Check sheet for the modelled part. Datum: model origin and axes. Units: mm. A direction names the side the tool comes from. Round coordinates to 2 decimals unless told otherwise and drop trailing zeros. Write each loop counter-clockwise with the first axis right and the second up, starting at its lowest first coordinate (ties: lowest second). Pieces come first, ordered by that corner, then holes. Notation, with made-up numbers: (-4, 33.25) - (42, 33.25) arc R21 ccw to (42, 67.25) - close; hole circle Ø11 at (85, 65.5). An arc over 180 degrees is marked (long way). Answer as a JSON object with one key per item and string values. Group by question number.
Item 1: Set-up check for faces 1 (the flat face through (-1.22, 0.49, -0.87)), 2 (the flat face through (0, 2, 0)), 3 (the cylindrical face through (-0.862, -0.596, 2.685)): record each of +Z, -Z, +X, -X, +Y, -Y from which the full face is reachable in a straight line by a thin tool's end or side.
Item 2: Sectioned sample at A-A on x = 5.75. Record the boundary of the cut face in (y, z), plus the area to 3 significant figures.
Item 3: Thickness scan on line 1 (X direction, y = 1.8, z = -0.9); line 2 (Z direction, x = -0.75, y = -0.5); line 3 (Y direction, x = 7.75, z = -1.15). Record the ranges inside material, lowest first.
Item 4: Release check for a two-part mould opening along Y. For faces 4 (the flat face through (10, 0, 0)), 5 (the flat face through (-1, -1, 0)), 6 (the cylindrical face through (4.83, -1.5, -0.07)) record: pulls with the +Y half, pulls with the -Y half, needs draft (parallel to the pull), parting line crosses it, or undercut.
Item 5: Gauge pin test, flat end, axial feed: P1, Ø3, axis at x = 3, z = -1, coming from the -Y side. Record the tip position at first contact, or that the pin passes through.
Autodesk Inventor part; units mm, degrees
ref_plane "Work Plane1" through (29, 0, 0) normal (0, -1, 0) x (1, 0, 0)
ref_plane "YZ Plane" through (0, 0, 0) normal (1, 0, 0) x (0, 1, 0)
ref_plane "XZ Plane" through (0, 0, 0) normal (0, 1, 0) x (-1, 0, 0)
sketch "Skizze1" plane through (0, 0, 0) normal (0, 0, 1) x (1, 0, 0)
  line L0 (0.1667, 0) -> (10, 0)
  line L1 (10, 0) -> (10, 1.5)
  line L2 (10, 1.5) -> (1.5, 1.5)
  line L3 (1.5, 1.5) -> (1.1932, 1.5)
  line L4 (1.1932, 1.5) -> (0, 1.5)
  line L5 (0, 1.5) -> (0, 2.75)
  line L6 (0, 2.75) -> (-2, 2.75)
  line L7 (-2, 2.75) -> (-2, 1.1547)
  line L8 (-2, 1.1547) -> (-0.5, 1.1547)
  line L9 (-0.5, 1.1547) -> (0.1667, 0)
  line L10 (-4.4, 0) -> (12.4, 0)
  line L11 (0, -0.55) -> (0, 3.3)
  line L12 (1.5, 1.5) -> (0, 1.5) construction
  dimension "d1" = 8.5
  dimension "d2" = 0.3068
  dimension "d3" = 2
  dimension "d4" = 1.5
  dimension "d5" = 60
  dimension "d6" = 3
  dimension "d7" = 3
  dimension "d8" = 2.3094
  dimension "d9" = 5.5
  dimension "d26" = 10
revolve "Körper" add sketch "Skizze1" angle 360 about axis through (0.1667, 0, 0) along (1, 0, 0) contours L9 L11 L4 L3 L2 L1 L0 | L9 L8 L7 L6 L5 L11
sketch "Skizze2" plane through (-2, 0, 0) normal (-1, 0, 0) x (0, 0, 1)
  circle A0 centre (0, 0) radius 1.1547
  line L0 (0, -3.85) -> (0, 3.85)
  line L1 (-3.85, 0) -> (3.85, 0)
  line L2 (1.1547, 0) -> (0.5774, -1)
  line L3 (0.5774, -1) -> (-0.5774, -1)
  line L4 (-0.5774, -1) -> (-1.1547, 0)
  line L5 (-1.1547, 0) -> (-0.5774, 1)
  line L6 (-0.5774, 1) -> (0.5774, 1)
  line L7 (0.5774, 1) -> (1.1547, 0)
  point P0 (0, 0)
extrude "Loch" add sketch "Skizze2" against normal up to next contours L7 A0 | A0 L2 | L6 L0 A0 | A0 L0 L3 | L0 L6 A0 | A0 L3 L0 | L4 A0 | A0 L5
fillet "Rundung1" radius 0.3 1 edges at (-2, -2.75, 0)
thread "Gewinde"
chamfer "Fase1" distance 0.3067 distance2 0.3067 1 edges at (10, -1.5, 0) measured on face at (10, -0.6587, -0.1791)
ref_plane "Work Plane1" through (29, 0, 0) normal (0, -1, 0) x (1, 0, 0)
fillet "Fillet2" radius 0.1 1 edges at (0, -1.5, 0)
equation "\"d1\" = GEL"
equation "\"d3\" = KOH"
equation "\"d4\" = INTI"
equation "\"d6\" = GD"
equation "\"d7\" = BDM"
equation "\"d8\" = 1.1547 * SW"
equation "\"d9\" = KOD"
equation "\"d26\" = NLG"
equation "\"d30\" = R"
equation "\"d17\" = RR"
equation "\"d13\" = GEL"
equation "\"d15\" = -0.5 * SPD + 0.5 * GD"
equation "\"d16\" = GUL"
equation "\"GD\" = NND"
equation "\"NLG\" = 10"
equation "\"GEL\" = 8.5"
equation "\"KOD\" = 5.5"
equation "\"KOH\" = 2"
equation "\"INTI\" = 1.5"
equation "\"GAL\" = 0.61345 * PTC"
equation "\"GUL\" = 0.61345 * PTC"
equation "\"BDM\" = NND"
equation "\"SW\" = 2"
equation "\"RR\" = 0.3"
equation "\"SPD\" = NND - 1.2269 * PTC"
equation "\"R\" = 0.1"
equation "\"TOA\" = 30deg"
equation "\"GD1\" = THREADDIA - 1.2269 * PTC"
equation "\"THREADDIA\" = 3"
equation "\"FAWI\" = 45deg"
equation "\"ANG\" = 120deg"
equation "\"PTC\" = 0.5"
equation "\"NND\" = 3"
equation "\"E0\" = 1.155 * SW"
properties part number "DIN 7984 - M3 x 10" material "Stahl, weich"
Completed:
{
 "1": {"face 1": "-X", "face 2": "+X", "face 3": "+X, -X"},
 "2": {"outline": "circle Ø3 at (0, 0)", "area": "7.07 mm²"},
 "3": {"line 1": "-2 to 0", "line 2": "-2.7 to -0.87, 0.87 to 2.7", "line 3": "-0.96 to 0.96"},
 "4": {"face 4": "needs draft", "face 5": "undercut", "face 6": "parting line crosses it"},
 "5": {"P1": "y = -1.5"}
}
